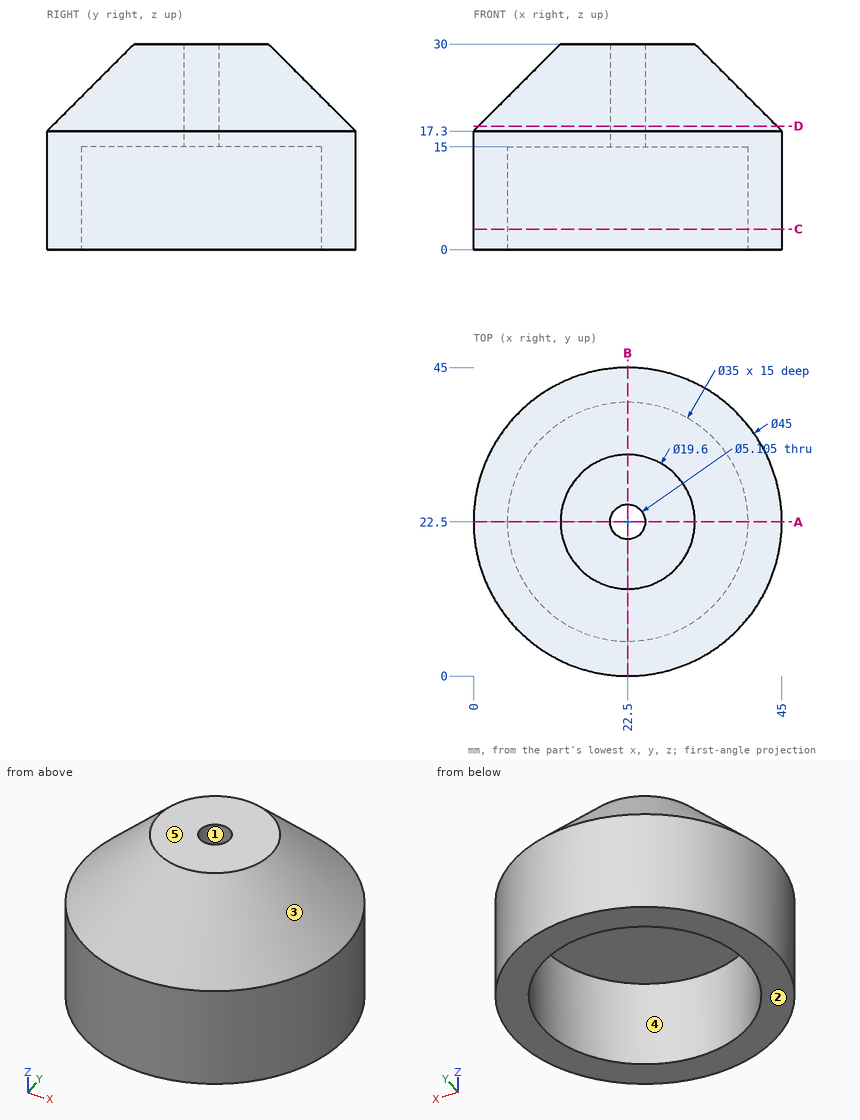
Study the drawing (mm; zero at the part's minimum x, y, z) and answer. A direction names the side the tool comes from. Give positions to 0.01 mm unless a question says otherwise; leave off trailing zeros. Loops run counter-clockwise (first coordinate to the right, second up) from the corner with the lowest first, then second, coordinate; pieces in that order, holes last. Notation, with made-up numbers: (33.25, 44.5) -> (41.25, 44.5) arc R23 ccw to (41.25, 68.5) -> close; hole circle Ø10 at (88, 20.5). An arc over 180 degrees is marked (long way). Write item = value, one per line. Start each with the question number.
(1) Find the intervals of material crossed by probe 1 along Y at (x, z) = (22.5, 7); probe 2 along Z at (x, y) = (32, 20.5); probe 3 along Y at (x, z) = (8.5, 14.25) (1 decimal), in increasing order. Write a range as from..to.
(2) The mould has two halves that part along X. Classify the marked faces 1, 2 and 3: +X half, -X half, draft (parallel to the pull), parting line (faces both ways), or undercut.
(3) Find section A-A on y = 22.5. Give the vertices of the cut face in (x, z).
(4) Given pin 1 Ø12 at (x, z) = (39, 24) entering from +Y; pin 2 Ø3 at (y, z) = (9.5, 9.5) entering from +X; pin 3 Ø12 at (x, z) = (35.5, 24) entering from +Y, each flat-ended and moving along its own axis, determine where each tip first touches the part or whether it passes through.
(5) Find section C-C on z = 3. Give the vertices of the cut face in (x, y).
(6) Find section D-D on z = 18. Give the vertices of the cut face in (x, y) (1 decimal).
(7) Which of the six approach directions +Z, -Z, +X, -X, +Y, -Y give full straight-line access (tool end or side, diameter ignored) to the marked faces 4 and 5?
From the geometry:
q1.probe_1 = 0..5, 40..45
q1.probe_2 = 15..30
q1.probe_3 = 4.9..12, 33..40.1
q2.face_1 = undercut
q2.face_2 = draft
q2.face_3 = parting line
q3.outline = (0, 0) -> (5, 0) -> (5, 15) -> (19.95, 15) -> (19.95, 30) -> (12.7, 30) -> (0, 17.3) -> close; (25.05, 15) -> (40, 15) -> (40, 0) -> (45, 0) -> (45, 17.3) -> (32.3, 30) -> (25.05, 30) -> close
q4.pin_1 = 38.59
q4.pin_2 = 41.84
q4.pin_3 = 40.98
q5.outline = circle Ø45 at (22.5, 22.5); hole circle Ø35 at (22.5, 22.5)
q6.outline = circle Ø43.6 at (22.5, 22.5); hole circle Ø5.1 at (22.5, 22.5)
q7.face_4 = -Z
q7.face_5 = +Z, +X, -X, +Y, -Y
